Geometry check sheet. Reference: the model listing, model coordinates, mm. Face numbers are marked on the shaded views. A direction names the side the tool comes from. Round coordinates to 2 decimals unless told otherwise and drop trailing zeros. Order: outer loops, then holes, each group sorted by start corner. A loop starts at its lowest first (then second) coordinate and runs counter-clockwise, first axis right, second up.
(1) Sectioned sample at C-C (x = 63.5). Record the boundary of the cut face in (y, z).
(2) Material ranges on line 1 along X through (y, z) = (-10.25, 64); line 2 along X through (y, z) = (-9.5, 63); line 3 along X through (y, z) = (-16.75, 20.5), recorded low to high.
(3) Release check for a two-part mould opening along X. For the marked faces 3, 4 and 5 record: +X half, -X half, draft (parallel to the pull), parting line (faces both ways), or undercut.
(4) Set-up check for the marked faces 1 and 2: record each of +Z, -Z, +X, -X, +Y, -Y from which the full face is reachable in a straight line by a thin tool's end or side.
(5) Sectioned sample at B-B (x = 0). Record the boundary of the cut face in (y, z).
(6) Go/stop test with flat-tipped pins: pin 1 (1.5 mm diameter, centred on x = 22, y = -11.5, fed in from +Z); pin 2 (9 mm diameter, centred on y = -8.5, z = 86, fed in from +X); pin 3 (2.5 mm diameter, centred on y = -10, z = 83.5, fed in from -X); pin 4 (6.5 mm diameter, centred on x = -2.5, z = 76.5, fed in from -Y). Record where each tip stops, or that it passes through.
(7) Sectioned sample at A-A (z = 24). Record the boundary of the cut face in (x, y).
from build123d import *

# Parameters (mm, degrees)
F1_DEPTH = 20
F2_DEPTH = 5
F4_R     = 3
F5_SIZE  = 2.99999
F6_W     = 80
F6_H     = 15
F7_DEPTH = 20
F8_R     = 5


# Not quite as in the source:
# - a fillet or chamfer is up to 0.001 mm smaller than in the source, because OpenCascade refuses the exact size
# - a pattern or mirror of a feature is missing from the dataset's text; its kind, count and spacing are read off the source's solid


with BuildPart() as f1:
    # F0 (on Front) → F1 (new body)
    with BuildSketch(Plane.XZ):
        with BuildLine():
            Line((-86.6025403784, -50), (86.6025403784, -50))
            ThreePointArc((86.6025403784, -50), (66.25695525, 31.4492148287), (10, 93.7635182946))
            Line((10, 93.7635182946), (10, 80))
            ThreePointArc((10, 80), (0, 70), (-10, 80))
            Line((-10, 80), (-10, 93.7635182946))
            ThreePointArc((-10, 93.7635182946), (-66.25695525, 31.4492148287), (-86.6025403784, -50))
        make_face()
        with BuildLine():
            ThreePointArc((20.8128184267, 66.1498526475), (55.1784519137, 20.1925765445), (70.8898326981, -35))
            Line((70.8898326981, -35), (-70.8898326981, -35))
            ThreePointArc((-70.8898326981, -35), (-55.1784519137, 20.1925765445), (-20.8128184267, 66.1498526475))
            ThreePointArc((-20.8128184267, 66.1498526475), (0, 55.000000149), (20.8128184267, 66.1498526475))
        make_face(mode=Mode.SUBTRACT)
    extrude(amount=F1_DEPTH)

    # F0 (on Front) → F2 (join)
    with BuildSketch(Plane.XZ):
        with BuildLine():
            ThreePointArc((-10, 80), (0, 70), (10, 80))
            Line((10, 80), (7, 80))
            ThreePointArc((7, 80), (0, 73), (-7, 80))
            Line((-7, 80), (-10, 80))
        make_face()
    f2 = extrude(amount=F2_DEPTH)

    # F2_copies: F2 across plane
    add(f2.mirror(Plane(origin=(0, -10, 0), x_dir=(0, 0, -1), z_dir=(0, -1, 0))))

    # F4
    f4_edges = [f1.edges().sort_by_distance(p)[0] for p in [
        (-10, -10, 93.763518),
        (10, -10, 93.763518),
        (86.60254, -10, -50),
        (-86.60254, -10, -50),
        (-70.889833, -10, -35),
        (70.889833, -10, -35),
        (20.812818, -10, 66.149853),
        (-20.812818, -10, 66.149853),
    ]]
    fillet(f4_edges, radius=F4_R)

    # F5 (size 3 in the source; OpenCascade refuses exactly that, so slightly less here)
    f5_edges = [f1.edges().sort_by_distance(p)[0] for p in [
        (-10, -2.5, 80),
        (-10, -10, 80),
        (-10, -17.5, 80),
        (10, -2.5, 80),
        (10, -10, 80),
        (10, -17.5, 80),
    ]]
    chamfer(f5_edges, length=F5_SIZE)

    # F6 (on face) → F7 (cut, through all)
    with BuildSketch(Plane(origin=(0, 0, 0), x_dir=(-1, 0, 0), z_dir=(0, 1, 0))):
        with Locations((0, -42.5)):
            Rectangle(F6_W, F6_H)
    extrude(amount=-F7_DEPTH, mode=Mode.SUBTRACT)

    # F8
    f8_edges = [f1.edges().sort_by_distance(p)[0] for p in [
        (40, -10, -35),
        (-40, -10, -35),
    ]]
    fillet(f8_edges, radius=F8_R)


solid = f1.part
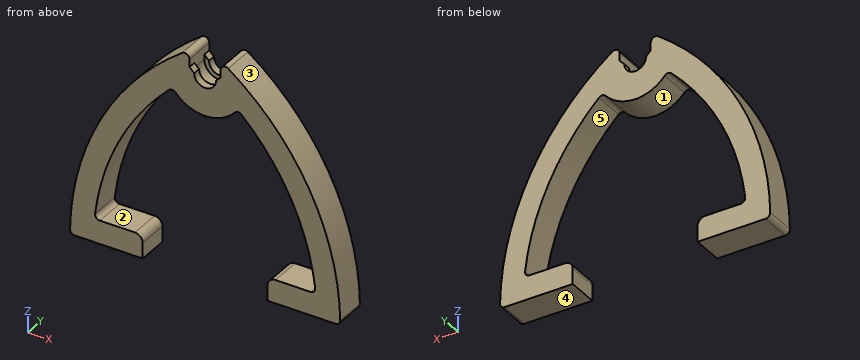
Answer below:
1. outline: (-20, -50) - (0, -50) - (0, -35) - (-20, -35) - close; (-20, -0.02) - (0, -0.02) - (0, 36.42) - (-20, 36.42) - close
2. line 1: x = -43.8 to -23.08, -19.27 to 19.27, 23.08 to 43.8
2. line 2: x = -44.66 to -24.12, -18.33 to 18.33, 24.12 to 44.66
2. line 3: x = -71.61 to -55.03, 55.03 to 71.61
3. face 3: +X half
3. face 4: draft
3. face 5: undercut
4. face 1: -Z, +Y, -Y
4. face 2: +Y, -Y
5. outline: (-20, 55) - (0, 55) - (0, 73) - (-5, 73) - (-5, 70) - (-15, 70) - (-15, 73) - (-20, 73) - close
6. pin 1: stops at z = 85.53
6. pin 2: stops at x = 26.13
6. pin 3: stops at x = -25.25
6. pin 4: stops at y = -20
7. outline: (-70, -20) - (-53.23, -20) - (-53.23, 0) - (-70, 0) - close; (53.23, -20) - (70, -20) - (70, 0) - (53.23, 0) - close
